Answer from the drawing. Dimensions are ordinates in mm from the lowest x, y and z of the part. A direction names the side the tool comes from. Coordinates: 2 decimals unless noted, no trailing zeros. Loops run counter-clockwise (first coordinate to the right, second up) from the corner with the lowest first, then second, coordinate; pieces in that order, holes last. Notation, with made-up numbers: M -27.5,9.5 L 8.5,9.5 A21 cw 8.5,44.5 Z; hole C 83,63 d1. An arc over 180 degrees is marked long. One line per item, written item: value. Start each with the question number.
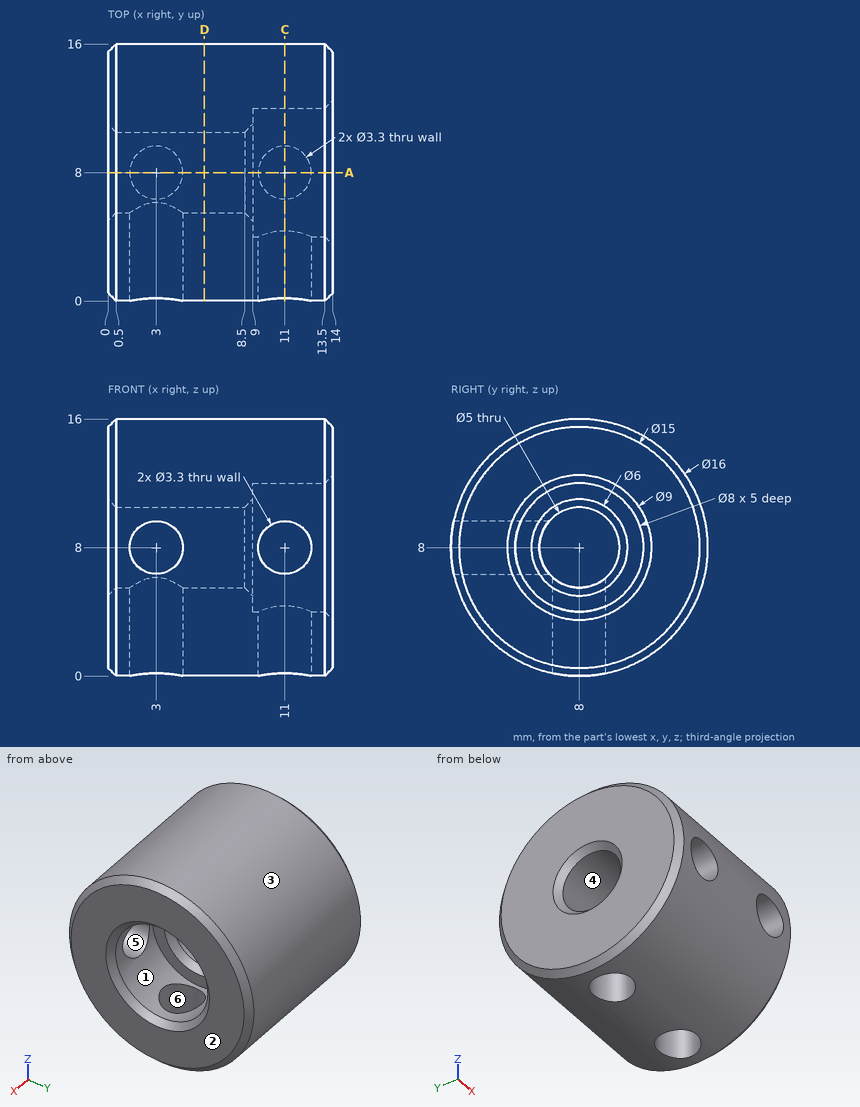
1) Section A-A (y = 8) is taken. Count the separate pieces of the cut face and the enclosed holes in it, then the cut area to 3 significant figures.
2) Section D-D (x = 6) is taken. Determine the outline of the cut face in (y, z).
3) A tool of negligible diameter and unlimited length cuts with its end or side. For the marked faces 4, 5 and 6, from which of +Z, -Z, +X, -X, +Y, -Y can it reach the whole face along a straight path? Write none if from no direction.
4) For a pull along Z with two mould halves and no side action, classify the marked faces 1, 2 and 3 as released by +Z, released by -Z, zero draft, split by the parting line, or undercut.
5) Section C-C (x = 11) is taken. Determine the outline of the cut face in (y, z).
6) Flat-ended cylindrical pins translate along their axes: pin 1 (2 mm diameter, centred on x = 3, y = 8, fed in from -Z); pin 2 (2 mm diameter, centred on x = 2.5, z = 2.5, fed in from -Y); pin 3 (6 mm diameter, centred on x = 6, z = 4.5, fed in from +Y). Find the tip coordinate at first contact, or state that the pin passes through.
7) Consider line 1 along Y through (x, z) = (8, 8); line 2 along Y through (x, z) = (4.5, 9.5); line 3 along X through (y, z) = (2.5, 6.5). Determine where each line is inside the solid, lowest interval first.
Results found:
1. separate pieces: 4
1. enclosed holes: 0
1. area: 106 mm²
2. outline: C 8,8 d16; hole C 8,8 d5
3. face 4: +X, -X
3. face 5: -Y
3. face 6: -Z
4. face 1: undercut
4. face 2: zero draft
4. face 3: split by the parting line
5. outline: M 0.17,6.35 A8 ccw 6.35,0.17 L 6.35,4.36 A4 cw 4.36,6.35 Z; M 0.17,9.65 L 4.36,9.65 A4 cw long 9.65,4.36 L 9.65,0.17 A8 ccw long Z
6. pin 1: stops at z = 10.29
6. pin 2: stops at y = 1.39
6. pin 3: stops at y = 15.98
7. line 1: y = 0 to 5.5, 10.5 to 16
7. line 2: y = 0.14 to 6, 10 to 15.86
7. line 3: x = 0 to 2.31, 3.69 to 10.31, 11.69 to 14
